Autodesk Inventor part; units mm, degrees
ref_plane "YZ Plane" through (0, 0, 0) normal (1, 0, 0) x (0, 1, 0)
ref_plane "XZ Plane" through (0, 0, 0) normal (0, 1, 0) x (-1, 0, 0)
ref_plane "XY Plane" through (0, 0, 0) normal (0, 0, 1) x (1, 0, 0)
sketch "Sketch1" plane through (0, 0, 0) normal (0, 1, 0) x (-1, 0, 0)
  line L0 (4.2489, -4.8935) -> (8.8452, -1.0368)
  line L1 (-0.6227, -5.5713) -> (0.8666, -5.5713)
  arc A0 (2.3695, -5.5775) -> (4.2489, -4.8935) centre (2.3418, -2.5777) ccw
  line L2 (0.8803, -5.5773) -> (2.3695, -5.5775)
  arc A1 (-2.502, -4.8873) -> (-0.6227, -5.5713) centre (-0.595, -2.5715) ccw
  circle A2 centre (6.3667, 0.9564) radius 1.55
  arc A3 (8.8452, -1.0368) -> (8.8476, 2.8817) centre (7.2935, 0.9234) ccw
  line L3 (-0.1334, 0.9212) -> (1.8666, 0.9212)
  arc A4 (-0.6442, 7.4287) -> (-2.5236, 6.7446) centre (-0.6165, 4.4288) ccw
  line L4 (-0.6442, 7.4287) -> (-0.1334, 7.4287)
  line L5 (-0.1334, 0.9212) -> (-0.1334, 7.4287)
  line L6 (1.8666, 0.9212) -> (1.8827, 7.4237)
  line L7 (1.8827, 7.4237) -> (2.372, 7.4225)
  arc A5 (4.2514, 6.7384) -> (2.372, 7.4225) centre (2.3443, 4.4226) ccw
  line L8 (4.2514, 6.7384) -> (8.8476, 2.8817)
  line L9 (-2.502, -4.8873) -> (-7.0983, -1.0306)
  line L10 (-2.5236, 6.7446) -> (-7.1199, 2.8879)
  circle A6 centre (-4.6336, 0.9477) radius 1.55
  arc A7 (-7.1199, 2.8879) -> (-7.0983, -1.0306) centre (-5.5563, 0.9372) ccw
  line L11 (0.8803, -5.5773) -> (0.8666, -5.5713)
  point P0 (0, 0)
  dimension "d0" = 2
  dimension "d1" = 3
  dimension "d2" = 2
  dimension "d3" = 3
  dimension "d4" = 2
  dimension "d5" = 3
  dimension "d6" = 2
  dimension "d7" = 3
  dimension "d8" = 3.1
  dimension "d9" = 3.1
  dimension "d10" = 6
  dimension "d11" = 6
  dimension "d12" = 2.5
  dimension "d13" = 6
  dimension "d14" = 6
  dimension "d15" = 2.5
extrude "Extrusion1" add sketch "Sketch1" along normal blind 2
properties part number "back_lock"
Design review of the part built by this model. Coordinates are the model's own, in mm. A direction names the side the tool comes from. Coordinates: 2 decimals unless noted, no trailing zeros. Order: outer loops, then holes, each group sorted by start corner. A loop starts at its lowest first (then second) coordinate and runs counter-clockwise, first axis right, second up. Notation, with made-up numbers: (-35, -25) -> (19, -25) arc R15 ccw to (19, -17) -> close; hole circle Ø8 at (5.5, -32.5). An arc over 180 degrees is marked (long way). One line per item, written item: value. Start each with the question number.
Q1. Take a section at A-A, the plane z = 4. State the section outline as (x, y) points.
Q2. Mouldability with a two-part tool opening along Z and no side actions: class faces 1 (the cylindrical face through (-9.793, 0.986, 0.953)), 2 (the flat face through (-1, 2, 0)), 3 (the cylindrical face through (6.182, 0.986, 0.88)) as pulls with the +Z half, pulls with the -Z half, needs draft (parallel to the pull), parting line crosses it, or undercut.
Q3. Take a section at B-B, the plane x = -7.5. State the section outline as (y, z) points, then the cut area to 3 significant figures.
Q4. For probe 1 along X at (y, z) = (0.5, 0.25); probe 2 along X at (y, z) = (1.65, 1.5); probe 3 along X at (y, z) = (0.75, 1.25), list the stretches that pass through material, from the lowest coordinate up.
Q5. Take a section at D-D, the plane x = -0.25. State the section outline as (y, z) points.
Q6. Tool access review of faces 4 (the flat face through (-1, 1, 0.921)), 5 (the flat face through (-1, 0, 0)): name each direction out of +Z, -Z, +X, -X, +Y, -Y from which nothing blocks a thin tool from reaching the whole face with its end or side.
Q7. Insertion check: pin 1 Ø1 at (y, z) = (1, 3.5) entering from +X; pin 2 Ø0.7 at (x, y) = (0, 0.5) entering from -Z; pin 3 Ø5 at (x, z) = (-2, 1.5) entering from -Y; pin 4 Ø1.9 at (x, z) = (-6.37, 0.96) entering from -Y. Each pin has a flat end and moves straight along its axis. Give the tip position at first contact, or say it passes through.
Q8. Take a section at C-C, the plane y = 0.95. Give the number of separate pieces and of enclosed holes in the cut face, then the cut area to 3 significant figures.
Values follow:
1. outline: (-7.51, 0) -> (-1.87, 0) -> (-1.87, 2) -> (-7.51, 2) -> close; (0.13, 0) -> (5.79, 0) -> (5.79, 2) -> (0.13, 2) -> close
2. face 1: parting line crosses it
2. face 2: needs draft
2. face 3: undercut
3. outline: (0, -2.17) -> (2, -2.17) -> (2, -0.1) -> (0, -0.1) -> close; (0, 2.01) -> (2, 2.01) -> (2, 4.01) -> (0, 4.01) -> close
3. area: 8.13 mm2
4. probe 1: x = -9.7 to -7.75, -4.99 to 3.25, 6.02 to 7.96
4. probe 2: x = -9.73 to -7.82, -4.92 to -1.87, 0.13 to 3.19, 6.08 to 7.99
4. probe 3: x = -9.77 to -7.89, -4.84 to -1.87, 0.13 to 3.11, 6.15 to 8.04
5. outline: (0, -5.57) -> (2, -5.57) -> (2, 0.92) -> (0, 0.92) -> close
6. face 4: +Z, +Y, -Y
6. face 5: +Z, -Z, +X, -X, -Y
7. pin 1: stops at x = 6.99
7. pin 2: stops at z = -5.57
7. pin 3: stops at y = 0
7. pin 4: passes through
8. separate pieces: 1
8. enclosed holes: 2
8. area: 135 mm2
